Design review of the part built by this model. Coordinates are the model's own, in mm. A direction names the side the tool comes from. Coordinates: 2 decimals unless noted, no trailing zeros. Write each loop counter-clockwise with the first axis right and the second up, starting at its lowest first coordinate (ties: lowest second). Pieces come first, ordered by that corner, then holes. Notation, with made-up numbers: M 23,55 L 30,55 A10 cw 30,62 Z; hole C 51,-0.5 d2. An arc over 180 degrees is marked long. Write item = value, one per line.
Autodesk Inventor part; units mm, degrees
ref_plane "Work Plane2" through (178, -56.0619, -70.2985) normal (1, 0, 0) x (0, 0.8411785, -0.5407576)
ref_plane "YZ Plane" through (0, 0, 0) normal (1, 0, 0) x (0, 1, 0)
ref_plane "XZ Plane" through (0, 0, 0) normal (0, 1, 0) x (-1, 0, 0)
ref_plane "Work Plane1" through (0, 4.7283, -22.9522) normal (-1, 0, 0) x (0, -0.8411785, 0.5407576)
sketch "Sketch1" plane through (0, 4.7283, -22.9522) normal (-1, 0, 0) x (0, -0.8411785, 0.5407576)
  line L0 (-61.5, -16.75) -> (-59.949, -16.75)
  line L1 (61.5, -12.25) -> (61.5, -16.75)
  line L2 (61.5, -16.75) -> (65.5, -16.75)
  line L3 (65.5, -16.75) -> (65.5, -20.25)
  line L4 (65.5, -20.25) -> (79.5, -20.25)
  line L5 (79.5, -20.25) -> (65.5, -11.25)
  line L6 (65.5, -11.25) -> (65.5, -12.25)
  line L7 (65.5, -12.25) -> (61.5, -12.25)
  line L8 (16.3889, 16.75) -> (16.3889, 18.75)
  line L9 (14.3494, 18.75) -> (16.3889, 18.75)
  line L10 (65.1985, -12.25) -> (12.6206, 21.5501)
  line L11 (16.3889, 16.75) -> (16.3889, 19.1276)
  arc A0 (-61.5, -15.199) -> (-59.949, -16.75) centre (-58.75, -14) ccw
  line L12 (-61.5, -15.199) -> (-61.5, -16.75)
  arc A1 (-57.551, -16.75) -> (-61.5, -12.801) centre (-58.75, -14) ccw
  line L13 (-57.551, -16.75) -> (-36.699, -16.75)
  arc A2 (-34.301, -16.75) -> (-36.699, -16.75) centre (-35.5, -14) ccw
  line L14 (-34.301, -16.75) -> (61.5, -16.75)
  line L15 (61.5, -16.75) -> (61.5, -12.25)
  line L16 (61.5, -12.25) -> (16.3889, 16.75)
  line L17 (16.3889, 16.75) -> (-61.5, 16.75)
  line L18 (-61.5, 16.75) -> (-61.5, -12.801)
  dimension "d14" = 2
ref_plane "Work Plane2" through (178, -56.0619, -70.2985) normal (1, 0, 0) x (0, 0.8411785, -0.5407576)
extrude "Extrusion1" add sketch "Sketch1" against normal up to surface (178 mm away) contours L16 L8 L11 L10 L7
sketch "Sketch2" plane through (0, -56.7396, 2) normal (0, 0, 1) x (1, 0, 0)
  circle A0 centre (3, 22.7682) radius 2.5
  circle A1 centre (3, 42.0825) radius 2.5
  line L0 (0, 3.1111) -> (0, 56.7396)
  line L1 (0, 3.1111) -> (6, 3.1111)
  line L2 (6, 56.7396) -> (6, 3.1111)
  line L3 (0, 56.7396) -> (6, 56.7396)
  circle A2 centre (175, 22.7682) radius 2.5
  circle A3 centre (175, 42.0825) radius 2.5
  line L4 (178, 3.1111) -> (178, 56.7396)
  line L5 (178, 56.7396) -> (172, 56.7396)
  line L6 (172, 56.7396) -> (172, 3.1111)
  line L7 (178, 3.1111) -> (172, 3.1111)
hole "Hole1" at (3, -14.6571, 2) at (3, -33.9713, 2) at (175, -33.9713, 2) at (175, -14.6571, 2) direction (0, 0, -1) diameter 3.6 end through all countersink diameter 7 countersink angle 90
ref_plane "Work Plane3" through (22, -30.5397, -9.0869) normal (0, -0.7712334, 0.6365525) x (1, 0, 0)
sketch "Sketch3" plane through (22, -30.5397, -9.0869) normal (0, -0.7712334, 0.6365525) x (1, 0, 0)
  line L0 (-9.9215, 5.4518) -> (-9.9215, -5.4534)
  spline S0 degree 3 poles (-9.9215, -5.4534) (-9.9222, -5.5772) (-9.8204, -5.8209) (-9.5772, -5.9222) (-9.4534, -5.9215) knots 0 0 0 0 0.5 1 1 1 1
  line L1 (-9.4534, -5.9215) -> (19.4534, -5.9215)
  spline S1 degree 3 poles (19.4534, -5.9215) (19.5775, -5.9222) (19.8219, -5.82) (19.9222, -5.5758) (19.9215, -5.4518) knots 0 0 0 0 0.5 1 1 1 1
  line L2 (19.9215, -5.4518) -> (19.9215, 5.4534)
  spline S2 degree 3 poles (19.9215, 5.4534) (19.9222, 5.5775) (19.82, 5.8219) (19.5758, 5.9222) (19.4518, 5.9215) knots 0 0 0 0 0.5 1 1 1 1
  line L3 (19.4518, 5.9215) -> (-9.4534, 5.9215)
  spline S3 degree 3 poles (-9.4534, 5.9215) (-9.5775, 5.9222) (-9.8219, 5.82) (-9.9222, 5.5758) (-9.9215, 5.4518) knots 0 0 0 0 0.5 1 1 1 1
  circle A0 centre (-8.3791, -4.3791) radius 0.5
  circle A1 centre (-8.3791, 4.3791) radius 0.5
  circle A2 centre (18.3791, 4.3791) radius 0.5
  circle A3 centre (18.3791, -4.3791) radius 0.5
  arc A4 (5.2617, -1.4512) -> (5.1811, -1.5218) centre (5.2771, -1.55) ccw
  arc A5 (5.1811, 1.5218) -> (5.1811, -1.5218) centre (0, 0) ccw
  arc A6 (5.1811, 1.5218) -> (5.2617, 1.4512) centre (5.2771, 1.55) ccw
  arc A7 (5.2617, 1.4512) -> (5.3414, 1.519) centre (5.2463, 1.55) ccw
  arc A8 (5.3414, -1.519) -> (5.3414, 1.519) centre (10, 0) ccw
  arc A9 (5.3414, -1.519) -> (5.2617, -1.4512) centre (5.2463, -1.55) ccw
  line L4 (143.9215, 5.4518) -> (143.9215, -5.4534)
  spline S4 degree 3 poles (143.4534, 5.9215) (143.5775, 5.9222) (143.8219, 5.82) (143.9222, 5.5758) (143.9215, 5.4518) knots 0 0 0 0 0.5 1 1 1 1
  line L5 (114.5482, 5.9215) -> (143.4534, 5.9215)
  spline S5 degree 3 poles (114.0785, 5.4534) (114.0778, 5.5775) (114.18, 5.8219) (114.4242, 5.9222) (114.5482, 5.9215) knots 0 0 0 0 0.5 1 1 1 1
  line L6 (114.0785, -5.4518) -> (114.0785, 5.4534)
  spline S6 degree 3 poles (114.5466, -5.9215) (114.4225, -5.9222) (114.1781, -5.82) (114.0778, -5.5758) (114.0785, -5.4518) knots 0 0 0 0 0.5 1 1 1 1
  line L7 (143.4534, -5.9215) -> (114.5466, -5.9215)
  spline S7 degree 3 poles (143.9215, -5.4534) (143.9222, -5.5772) (143.8204, -5.8209) (143.5772, -5.9222) (143.4534, -5.9215) knots 0 0 0 0 0.5 1 1 1 1
  circle A10 centre (142.3791, -4.3791) radius 0.5
  circle A11 centre (142.3791, 4.3791) radius 0.5
  circle A12 centre (115.6209, 4.3791) radius 0.5
  circle A13 centre (115.6209, -4.3791) radius 0.5
  arc A14 (128.8189, -1.5218) -> (128.7383, -1.4512) centre (128.7229, -1.55) ccw
  arc A15 (128.7383, -1.4512) -> (128.6586, -1.519) centre (128.7537, -1.55) ccw
  arc A16 (128.6586, 1.519) -> (128.6586, -1.519) centre (124, 0) ccw
  arc A17 (128.6586, 1.519) -> (128.7383, 1.4512) centre (128.7537, 1.55) ccw
  arc A18 (128.7383, 1.4512) -> (128.8189, 1.5218) centre (128.7229, 1.55) ccw
  arc A19 (128.8189, -1.5218) -> (128.8189, 1.5218) centre (134, 0) ccw
  circle A20 centre (10, 0) radius 5.4
  circle A21 centre (124, 0) radius 5.4
  line L8 (0, 5.4) -> (10, 5.4)
  line L9 (10, -5.4) -> (0, -5.4)
  line L10 (124, 5.4) -> (134, 5.4)
  line L11 (134, -5.4) -> (124, -5.4)
  point P0 (-22, 26.4483)
  dimension "d9" = 10.8
  dimension "d10" = 10.8
extrude "Extrusion2" cut sketch "Sketch3" along normal blind 78.25 contours A9 A8 A7 A6 A5 A20 A4 | A4 A5 A20 A6 A7 A8 A9 | A20 L9 A5 | A5 A20 | A5 L8 A20 | A19 A21 A18 A17 A16 A15 A14 | A14 A15 A16 A17 A18 A19 A21 | A21 A19 | A19 L11 A21 | A19 A21 L10
properties part number "front"
Q1. For P1, Ø4, axis at x = 3, y = -14.66, coming from the +Z side, flat-tipped, find the tip position at first contact; note if it passes through.
Check result:
P1 = 0.5
Q2. Consider section B-B, the plane x = 3. State the section outline as (y, z) points.
Check result:
outline = M -56.74,2 L -53.63,0 L -35.77,0 L -35.77,0.3 L -37.47,2 Z; M -32.17,0 L -16.46,0 L -16.46,0.3 L -18.16,2 L -30.47,2 L -32.17,0.3 Z; M -12.86,0 L 0,0 L 1.29,2 L -11.16,2 L -12.86,0.3 Z
Q3. Wall thickness on line 1 (X direction, y = -42.5, z = 0.95); line 2 (X direction, y = -46, z = 0.4); line 3 (Y direction, x = 3, z = 0.1): over which ranges is each line inside the solid? List them lowest first.
Check result:
line_1 = 0 to 16.6, 37.4 to 140.6, 161.4 to 178
line_2 = 0 to 17.23, 36.77 to 141.23, 160.77 to 178
line_3 = -53.78 to -35.77, -32.17 to -16.46, -12.86 to 0.06
Q4. Consider section A-A, the plane x = 154.5. State the section outline as (y, z) points, and give its area (3 significant figures).
Check result:
outline = M -56.74,2 L -53.63,0 L -50.03,0 L -52.46,2 Z; M -35.49,2 L -33.07,0 L 0,0 L 1.29,2 Z
area = 77.7 mm²
Q5. The part is to be moulded in two halves that separate along Y. For faces 3 (the flat face through (88, -27, 0)), 4 (the cylindrical face through (2.46, -35.69, 0.15)), 5 (the flat face through (87.754, -55.206, 1.014)), say which applies: +Y half, -Y half, draft (parallel to the pull), parting line (faces both ways), or undercut.
Check result:
face_3 = draft
face_4 = undercut
face_5 = -Y half
Q6. Machinability: for faces 1 (the cylindrical face through (161.4, -42.7, 1)), 2 (the conical face through (4.89, -14.409, 0.406)), which of the approach directions +Z, -Z, +X, -X, +Y, -Y give a long, thin tool a straight path to every point of the face, cutting with its end or side? Answer none if there is none.
Check result:
face_1 = none
face_2 = +Z
Q7. Consider section C-C, the plane z = 0.85. State how many separate pieces and enclosed holes the cut face has, and give its area (3 significant figures).
Check result:
separate_pieces = 1
enclosed_holes = 6
area = 9,180 mm²
